The listing builds one solid part. Answer for the finished solid, in the listing's coordinates (mm). A direction names the side the tool comes from. Coordinates: 2 decimals unless noted, no trailing zeros. Order: outer loops, then holes, each group sorted by start corner. A loop starts at its lowest first (then second) coordinate and runs counter-clockwise, first axis right, second up.
Autodesk Inventor part; units mm, degrees
ref_plane "Work Plane1" through (21.4313, 0, 10.922) normal (0, 0, 1) x (1, 0, 0)
ref_plane "YZ Plane" through (0, 0, 0) normal (1, 0, 0) x (0, 1, 0)
ref_plane "XZ Plane" through (0, 0, 0) normal (0, 1, 0) x (-1, 0, 0)
sketch "Sketch1" plane through (0, 0, 0) normal (0, 0, 1) x (1, 0, 0)
  line L0 (0, 0) -> (36.195, 0)
  line L1 (0, 7.9375) -> (10.414, 7.9375)
  line L2 (10.414, 7.9375) -> (10.414, 7.9248)
  line L3 (10.414, 7.9248) -> (12.7, 7.9248)
  line L4 (12.7, 7.9248) -> (12.7, 9.525)
  line L5 (12.7, 9.525) -> (30.1625, 9.525)
  line L6 (30.1625, 9.525) -> (30.1625, 10.922)
  line L7 (30.1625, 10.922) -> (34.163, 10.922)
  line L8 (34.163, 10.922) -> (34.163, 8.89)
  line L9 (34.163, 8.89) -> (36.195, 10.922)
  line L10 (36.195, 10.922) -> (36.195, 5.715)
  line L11 (0, 7.9375) -> (0, 4.445)
  line L12 (0, 3.175) -> (12.065, 3.175)
  line L13 (36.195, 5.715) -> (36.195, 0) construction
  line L14 (0, 3.175) -> (0, 0) construction
  line L15 (34.163, 10.922) -> (36.195, 10.922) construction
  line L16 (30.1625, 8.89) -> (34.163, 8.89) construction
  line L17 (12.7, 9.525) -> (12.7, 10.922)
  line L18 (12.7, 10.922) -> (30.1625, 10.922)
  circle A0 centre (25.4, 0) radius 4.7625
  line L19 (17.145, 3.175) -> (17.145, 5.715)
  line L20 (17.145, 5.715) -> (34.163, 5.715)
  line L21 (36.195, 10.3832) -> (34.163, 8.3512)
  line L22 (34.163, 8.3512) -> (34.163, 5.715)
  line L23 (34.163, 8.89) -> (34.163, 8.3512) construction
  line L24 (34.163, 5.715) -> (36.195, 5.715) construction
  line L25 (0, 4.445) -> (12.065, 4.445)
  line L26 (12.065, 4.445) -> (12.065, 3.175)
  line L27 (12.065, 3.175) -> (17.145, 3.175)
  line L28 (0, 4.445) -> (0, 3.175)
  dimension "d0" = 17.4625
  dimension "d2" = 15.8496
  dimension "d3" = 15.875
  dimension "d4" = 2.286
  dimension "d5" = 12.7
  dimension "d6" = 6.35
  dimension "d7" = 19.05
  dimension "d8" = 21.844
  dimension "d9" = 17.78
  dimension "d10" = 45
  dimension "d11" = 36.195
  dimension "d23" = 9.525
  dimension "d24" = 25.4
  dimension "d34" = 11.43
  dimension "d35" = 19.05
  dimension "d36" = 0.381
  dimension "d45" = 12.065
  dimension "d46" = 8.89
revolve "Revolution1" add sketch "Sketch1" angle 360 about axis through (0, 0, 0) along (1, 0, 0) contours L1 L2 L3 L4 L5 L6 L7 L8 L9 L10 L21 L22 L20 L19 L27 L26 L25 L11 | L17 L18 L6 L5
extrude "Extrusion1" cut sketch "Sketch1" along normal through all both and the other way through all contours L17 L18 L6 L5
extrude "Extrusion2" cut sketch "Sketch1" along normal through all contours A0 L0 | L0 A0
thread "Thread1"
chamfer "Chamfer1" distance 0.508 angle 45 2 edges at (12.7, -7.9248, 0) (0, -7.9375, 0)
chamfer "Chamfer2" distance 0.762 angle 45 1 edges at (20.6375, 0.0005, 10.922)
pattern_circular "Circular Pattern1" count 2 over 360 about axis through (21.4313, 0, 0) along (1, 0, 0) of "Extrusion1"
thread "Thread3"
fillet "Fillet1" radius 0.0508 6 edges at (36.195, -10.922, 0) (34.163, -8.89, 0) (34.163, -10.922, 0) (30.1625, 10.567, 2.7621) (30.1625, 10.567, -2.7621) (30.1625, -10.922, 0)
ref_plane "Work Plane1" through (21.4313, 0, 10.922) normal (0, 0, 1) x (1, 0, 0)
sketch "Sketch2" plane through (21.4313, 0, 10.922) normal (0, 0, 1) x (1, 0, 0)
  circle A0 centre (3.9687, 0.0595) radius 6.35
  line L0 (3.9687, 0.0595) -> (3.9687, -4.7625) construction
  point P0 (-21.4313, 0)
  dimension "d41" = 12.7
  dimension "d44" = 4.822
extrude "Extrusion4" cut sketch "Sketch2" against normal blind 2.54
properties part number "Rebuild Shooter NCDME075-0600 Cylinder Front Section" material "Aluminum 6061"
1) Determine the mould class of faces 1 (the face through (12.7, -7, -5)), 2 (the face through (25.77, -1.24, -5.58)), 3 (the face through (17.145, 2.5, -2.5)), 4 (the face through (34.366, 8.673, 2.731)) for opening direction Z: released by +Z, released by -Z, zero draft, split by the parting line, or undercut.
2) Section C-C (x = 11) is taken. Give the vertices of the cut face in (y, z) (3 decimals), then the cut area to 3 significant figures.
3) A tool of negligible diameter and unlimited length cuts with its end or side. For faces 5 (the face through (21, 9.525, 0)), 6 (the face through (24.37, 4.65, 6.31)), 7 (the face through (34.163, 2, 9)), 8 (the face through (6.12, -0.96, -4.34)), from which of +Z, -Z, +X, -X, +Y, -Y can it reach the whole face along a straight path? Write none if from no direction.
4) Section A-A (x = 16.5) is taken. Give the vertices of the cut face in (y, z) (3 decimals), then the cut area to 3 significant figures.
5) Section B-B (x = 25.4) is taken. Give the vertices of the cut face in (y, z) (1 decimal).
6) Each of these flat-tipped pins is pushed along its axis until it touches: P1, Ø8.5, axis at y = -1.5, z = -1.5, coming from the +X side; P2, Ø4, axis at x = 25.5, z = 6, coming from the +Y side (3 decimals); P3, Ø5, axis at y = 0.5, z = -0.5, coming from the +X side (3 decimals). Where does it stop, or does it pass through?
7) Consider L1, parallel to X at y = 0, z = 6.85; L2, parallel to Z at x = 15.15, y = 0 (3 decimals); L3, parallel to Y at x = 28, z = 2 (3 decimals). Determine where each line is inside the solid, lowest interval first.
Filled sheet:
1. face 1: zero draft
1. face 2: undercut
1. face 3: undercut
1. face 4: split by the parting line
2. outline: circle Ø15.85 at (0, 0); hole circle Ø8.89 at (0, 0)
2. area: 135 mm2
3. face 5: +Z, -Z, -X, +Y
3. face 6: +Z
3. face 7: none
3. face 8: -X
4. outline: (-9.525, -5.345) arc R10.922 ccw to (9.525, -5.345) - (9.525, 5.345) arc R10.922 ccw to (-9.525, 5.345) - close; hole circle Ø6.35 at (0, 0)
4. area: 323 mm2
5. outline: (-9.5, -5.3) arc R10.9 ccw to (9.5, -5.3) - (9.5, 5.3) arc R10.9 ccw to (6.4, 8.8) - (6.4, 8.4) - (4.8, 8.4) - (4.8, 3.2) arc R5.7 cw (long way) to (-4.8, 3.2) - (-4.8, 8.4) - (-6.3, 8.4) - (-6.3, 8.9) arc R10.9 ccw to (-9.5, 5.3) - close
6. P1: stops at x = 34.16
6. P2: stops at y = 9.525
6. P3: stops at x = 17.145
7. L1: x = 0 to 20.64, 30.16 to 34.16
7. L2: z = -10.922 to -3.175, 3.175 to 10.922
7. L3: y = -9.525 to -5.354, 5.354 to 9.525
